Check sheet for the modelled part. Datum: model origin and axes. Units: mm. Face numbers are marked on the shaded views. Coordinates: 2 decimals unless noted, no trailing zeros. Loops run counter-clockwise (first coordinate to the right, second up) from the corner with the lowest first, then second, coordinate; pieces in that order, holes last. Notation, with made-up numbers: (-10.5, -18) - (43.5, -18) arc R12 cw to (43.5, 1) - close; hole circle Ø7 at (30.25, 87). An arc over 180 degrees is marked (long way). Write each question's results on one line, items separated by ' | '. Start each with the question number.
1. Gauge pin test, flat ends, axial feed: P1, Ø1.5, axis at x = -3, z = 2.5, coming from the -Y side; P2, Ø1, axis at x = 2, z = 1.5, coming from the +Y side. Record the tip position at first contact, or that the pin passes through.
2. Cross-section at B-B (x = 1.5). Record the cut outline in (y, z).
3. Cross-section at D-D (y = -17.5). Record the cut outline in (x, z), and give its area (3 significant figures).
4. Cross-section at A-A (z = 2.35). Record the cut outline in (x, y).
5. Cross-section at C-C (y = 18.5). Record the cut outline in (x, z).
6. Thickness scan on line 1 (Y direction, x = -1, z = 0.45); line 2 (X direction, y = 18.5, z = 2.85); line 3 (X direction, y = -16, z = 1.6). Record the ranges inside material, lowest first. Write a range as [from, to].
7. Draft check along Y on the marked faces 1, 2 and 3. Enter one of: released by +Y, released by -Y, zero draft, split by the parting line, or undercut.
```python
from build123d import *

# Parameters (mm, degrees)
F0_W        = 14.6192193359
F0_H        = 50
F0_R        = 2.5
F1_DEPTH    = 3.2
F2_T1_DEPTH = 43.2
F3_T1_DEPTH = 43.2


# Not quite as in the source:
# - a fillet or chamfer that OpenCascade refuses, or shapes differently, is made with other operations: its cross-section is extruded or revolved along the edge and cut away or added


with BuildPart() as f1:
    # F0 (on Top) → F1 (new body)
    with BuildSketch(Plane.XY):
        Rectangle(F0_W, F0_H)
        with Locations((0, -17.5)):
            Circle(F0_R, mode=Mode.SUBTRACT)
        with Locations((0, 17.5)):
            Circle(F0_R, mode=Mode.SUBTRACT)
    extrude(amount=F1_DEPTH)

    # F2: fillet of radius 8 on 2 edges, made by hand

    # F2_s2 → F2_t1 (cut)
    with BuildSketch(Plane.XY.offset(-20)):
        with BuildLine():
            ThreePointArc((-0.6903903321, -25), (4.9664639174, -22.6568542495), (7.3096096679, -17))
            Line((7.3096096679, -17), (7.3096096679, -25))
            Line((7.3096096679, -25), (-0.6903903321, -25))
        make_face()
        with BuildLine():
            ThreePointArc((0.6903903321, -25), (-4.9664639174, -22.6568542495), (-7.3096096679, -17))
            Line((-7.3096096679, -17), (-7.3096096679, -25))
            Line((-7.3096096679, -25), (0.6903903321, -25))
        make_face()
    extrude(amount=F2_T1_DEPTH, mode=Mode.SUBTRACT)

    # F3: fillet of radius 8 on 2 edges, made by hand

    # F3_s2 → F3_t1 (cut)
    with BuildSketch(Plane.XY.offset(-20)):
        with BuildLine():
            ThreePointArc((-0.6903903321, 25), (4.9664639174, 22.6568542495), (7.3096096679, 17))
            Line((7.3096096679, 17), (7.3096096679, 25))
            Line((7.3096096679, 25), (-0.6903903321, 25))
        make_face()
        with BuildLine():
            ThreePointArc((-7.3096096679, 17), (-4.9664639174, 22.6568542495), (0.6903903321, 25))
            Line((0.6903903321, 25), (-7.3096096679, 25))
            Line((-7.3096096679, 25), (-7.3096096679, 17))
        make_face()
    extrude(amount=F3_T1_DEPTH, mode=Mode.SUBTRACT)


solid = f1.part
```
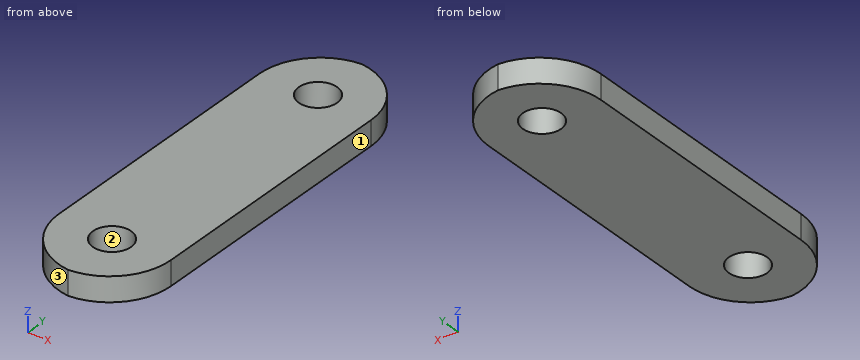
Established:
1) P1: y = -24.44 | P2: y = 24.69
2) outline: (-24.69, 0) - (-19.5, 0) - (-19.5, 3.2) - (-24.69, 3.2) - close; (-15.5, 0) - (15.5, 0) - (15.5, 3.2) - (-15.5, 3.2) - close; (19.5, 0) - (24.69, 0) - (24.69, 3.2) - (19.5, 3.2) - close
3) outline: (-7.29, 0) - (-2.5, 0) - (-2.5, 3.2) - (-7.29, 3.2) - close; (2.5, 0) - (7.29, 0) - (7.29, 3.2) - (2.5, 3.2) - close | area: 30.7 mm^2
4) outline: (-7.31, -17) arc R8 ccw to (0, -24.97) arc R8 ccw to (7.31, -17) - (7.31, 17) arc R8 ccw to (0, 24.97) arc R8 ccw to (-7.31, 17) - close; hole circle Ø5 at (0, -17.5); hole circle Ø5 at (0, 17.5)
5) outline: (-7.17, 0) - (-2.29, 0) - (-2.29, 3.2) - (-7.17, 3.2) - close; (2.29, 0) - (7.17, 0) - (7.17, 3.2) - (2.29, 3.2) - close
6) line 1: [-24.82, -19.79], [-15.21, 15.21], [19.79, 24.82] | line 2: [-7.17, -2.29], [2.29, 7.17] | line 3: [-7.31, -2], [2, 7.31]
7) face 1: zero draft | face 2: undercut | face 3: released by -Y
